Could you check a few things on this model? Use its own coordinates, in mm. A direction names the side the tool comes from. Give positions to 0.01 mm unless a question says otherwise; leave off trailing zeros. Loops run counter-clockwise (first coordinate to the right, second up) from the corner with the lowest first, then second, coordinate; pieces in that order, holes last.
1. For P1, Ø3, axis at x = 69, z = -1, coming from the -Y side, with a flat end and sliding along its axis, tell me the tip position at first contact or that it passes through.
2. Imagine slicing it at A-A (z = 0). List the corners of the cut face in (x, y) for me (3 decimals).
3. Thinking about a two-plate mould opening in X: for faces 3 (the flat face through (38, 0, -3.175)), 4 (the flat face through (-393.7, 2, -3)), 5 (the flat face through (6, -6.411, -4)), 6 (the flat face through (393.7, 2, 3)), which applies, +X half, -X half, draft (parallel to the pull), parting line (faces both ways), or undercut?
4. I need wall thicknesses on line 1 along Z through (x, y) = (63, -5.25) (3 decimals); line 2 along X through (y, z) = (5.75, 1.75); line 3 along X through (y, z) = (-1.5, 5). Which ranges of each line are inside material? Lowest first, please.
5. Imagine slicing it at B-B (y = 0). List the corners of the cut face in (x, z) for me (3 decimals).
6. For faces 1 (the flat face through (38, 0, 3.175)), 2 (the flat face through (6, 0, -6.35)), which set-ups out of +Z, -Z, +X, -X, +Y, -Y let a thin tool reach every point of the face, with its end or its side?
```python
from build123d import *

# Parameters (mm, degrees)
SKETCH1_W          = 12.7
SKETCH1_H          = 12.82133758
LENGTH_DEPTH       = 406.4
SKETCH2_W          = 12.7
SKETCH2_H          = 12.82133758
SKETCH2_R          = 3.175
ROUND_CUT_1_DEPTH  = 12.7
SKETCH3_W          = 12.7
SKETCH3_H          = 12.82133758
SKETCH3_R          = 3.175
ROUND_CUT_2_DEPTH  = 12.7
CUT_EXTRUDE1_REACH = 14.821
SKETCH5_W          = 76.2
SKETCH5_H          = 6.35


with BuildPart() as part:
    # Sketch1 → Length (new body, symmetric)
    with BuildSketch(Plane(origin=(0, 0, 0), x_dir=(0, 0, -1), z_dir=(1, 0, 0))):
        Rectangle(SKETCH1_W, SKETCH1_H)
    extrude(amount=LENGTH_DEPTH, both=True)

    # Sketch2 → Round Cut 1 (cut)
    with BuildSketch(Plane(origin=(406.4, 0, 0), x_dir=(0, 0, -1), z_dir=(1, 0, 0))):
        Rectangle(SKETCH2_W, SKETCH2_H)
        Circle(SKETCH2_R, mode=Mode.SUBTRACT)
    extrude(amount=-ROUND_CUT_1_DEPTH, mode=Mode.SUBTRACT)

    # Sketch3 → Round Cut 2 (cut)
    with BuildSketch(Plane.ZY.offset(406.4)):
        Rectangle(SKETCH3_W, SKETCH3_H)
        Circle(SKETCH3_R, mode=Mode.SUBTRACT)
    extrude(amount=-ROUND_CUT_2_DEPTH, mode=Mode.SUBTRACT)

    # Sketch5 → Cut-Extrude1 (cut, up to next)
    with BuildSketch(Plane(origin=(0, 6.41066879, 0), x_dir=(1, 0, 0), z_dir=(0, 1, 0)), mode=Mode.PRIVATE) as cut_extrude1_sk1:
        with Locations((38.1, 0)):
            Rectangle(SKETCH5_W, SKETCH5_H)
    cut_extrude1_tool1 = extrude(cut_extrude1_sk1.sketch, amount=-CUT_EXTRUDE1_REACH, mode=Mode.PRIVATE) & part.part
    add(cut_extrude1_tool1.solids().sort_by_distance((38.1, 6.410669, 0))[0], mode=Mode.SUBTRACT)


solid = part.part
```
Derived:
1. P1: passes through
2. outline: (-406.4, -3.175) - (-393.7, -3.175) - (-393.7, -6.411) - (0, -6.411) - (0, 6.411) - (-393.7, 6.411) - (-393.7, 3.175) - (-406.4, 3.175) - close; (76.2, -6.411) - (393.7, -6.411) - (393.7, -3.175) - (406.4, -3.175) - (406.4, 3.175) - (393.7, 3.175) - (393.7, 6.411) - (76.2, 6.411) - close
3. face 3: undercut
3. face 4: -X half
3. face 5: draft
3. face 6: +X half
4. line 1: z = -6.35 to -3.175, 3.175 to 6.35
4. line 2: x = -393.7 to 0, 76.2 to 393.7
4. line 3: x = -393.7 to 393.7
5. outline: (-406.4, -3.175) - (-393.7, -3.175) - (-393.7, -6.35) - (393.7, -6.35) - (393.7, -3.175) - (406.4, -3.175) - (406.4, 3.175) - (393.7, 3.175) - (393.7, 6.35) - (-393.7, 6.35) - (-393.7, 3.175) - (-406.4, 3.175) - close; hole (0, -3.175) - (76.2, -3.175) - (76.2, 3.175) - (0, 3.175) - close
6. face 1: +Y, -Y
6. face 2: -Z, +X, -X, +Y, -Y
